from build123d import *

# Parameters (mm, degrees)
SCHIZZO2_W               = 20.11559051
SCHIZZO2_H               = 2
TAGLIO_ESTRUSIONE1_DEPTH = 2


with BuildPart() as part:
    # Schizzo1 → Rivoluzione1 (revolve)
    with BuildSketch(Plane.XY):
        Polygon((0, 15), (2, 15), (2, 9), (1.409533837, 9), (1.409533837, 4.7), (7.5, 4.7), (7.5, 0), (0, 0), align=None)
    revolve(axis=Axis((0, -3.578292252, 0), (0, 1, 0)))

    # Schizzo2 → Taglio-Estrusione1 (cut)
    with BuildSketch(Plane.XZ):
        Rectangle(SCHIZZO2_W, SCHIZZO2_H)
    extrude(amount=-TAGLIO_ESTRUSIONE1_DEPTH, mode=Mode.SUBTRACT)


solid = part.part
Design review of the part built by this model. Coordinates are the model's own, in mm. A direction names the side the tool comes from. Give positions to 0.01 mm unless a question says otherwise; leave off trailing zeros. Loops run counter-clockwise (first coordinate to the right, second up) from the corner with the lowest first, then second, coordinate; pieces in that order, holes last. Notation, with made-up numbers: (85.5, -38) -> (100.5, -38) arc R31 cw to (100.5, -13) -> close; hole circle Ø10 at (-37, 43.5). An arc over 180 degrees is marked (long way). One line per question, with ' | ' between items. Start each with the question number.
(1) Draft analysis for pull direction Y (two halves, no side actions). For faces 5 (the face through (-0.306, 6.82, 1.376)), 6 (the face through (0, 0, 3)), 7 (the face through (0, 1, 1)), state which applies: +Y half, -Y half, draft (parallel to the pull), parting line (faces both ways), or undercut.
(2) We need section A-A (x = 0). State the section outline as (y, z) points.
(3) For line 1 (Y direction, x = 0, z = 2.5); line 2 (X direction, y = 0.75, z = -4); line 3 (X direction, y = 2.25, z = -3), list the stretches that pass through material, from the lowest coordinate up.
(4) We need section B-B (z = 0). State the section outline as (x, y) points, and give its area (3 significant figures).
(5) For faces 1 (the face through (0, 0, -4)), 2 (the face through (0.9, 9, 1.3)), 3 (the face through (0, 12, 2)), 4 (the face through (0, 1, -1)), list the 3-axis set-ups (+Z, -Z, +X, -X, +Y, -Y) from which the entire face can be reached by the end or side of a thin tool; tool diameter is ignored.
(6) Insertion check: P1, Ø6, axis at x = -1.5, y = 9.5, coming from the +Z side; P2, Ø3, axis at x = -4.5, z = -4.5, coming from the +Y side; P3, Ø1.6, axis at x = 2.5, y = 1, coming from the -Z side. Each pin has a flat end and moves straight along its axis. Give the tip position at first contact, or say it passes through.
(7) We need section D-D (x = -4.5). State the section outline as (y, z) points, and give its area (3 significant figures).
(8) We need section C-C (y = 9.75). State the section outline as (x, z) points, and give its area (3 significant figures).
The answers:
1) face 5: undercut | face 6: -Y half | face 7: draft
2) outline: (0, -7.5) -> (4.7, -7.5) -> (4.7, -1.41) -> (9, -1.41) -> (9, -2) -> (15, -2) -> (15, 2) -> (9, 2) -> (9, 1.41) -> (4.7, 1.41) -> (4.7, 7.5) -> (0, 7.5) -> (0, 1) -> (2, 1) -> (2, -1) -> (0, -1) -> close
3) line 1: y = 0 to 4.7 | line 2: x = -6.34 to 6.34 | line 3: x = -6.87 to 6.87
4) outline: (-7.5, 2) -> (7.5, 2) -> (7.5, 4.7) -> (1.41, 4.7) -> (1.41, 9) -> (2, 9) -> (2, 15) -> (-2, 15) -> (-2, 9) -> (-1.41, 9) -> (-1.41, 4.7) -> (-7.5, 4.7) -> close | area: 76.6 mm^2
5) face 1: +Z, -Z, +X, -X, -Y | face 2: none | face 3: +Y | face 4: +X, -X, -Y
6) P1: stops at z = 2 | P2: stops at y = 4.7 | P3: stops at z = -7.3
7) outline: (0, -6) -> (4.7, -6) -> (4.7, 6) -> (0, 6) -> (0, 1) -> (2, 1) -> (2, -1) -> (0, -1) -> close | area: 52.4 mm^2
8) outline: circle Ø4 at (0, 0) | area: 12.6 mm^2
